Design review of the part shown in the three views and the two pictorial views. Dimensions are in mm from the part's minimum x, y and z. Round coordinates to 2 decimals unless told otherwise and drop trailing zeros. Write each loop counter-clockwise with the first axis right and the second up, starting at its lowest first coordinate (ties: lowest second). Pieces come first, ordered by that corner, then holes. Notation, with made-up numbers: (45, -23.5) -> (90, -23.5) arc R22 cw to (90, -15.5) -> close; hole circle Ø8 at (-21.5, 56.25). An arc over 180 degrees is marked (long way). Answer as a JSON object with one key per item and string values. Group by question number.
1) We need section D-D, the plane x = 56. Write out the cut boundary in (y, z), then the cut area to 3 significant figures.
2) We need section C-C, the plane x = 26.5. Write out the cut boundary in (y, z), then the cut area to 3 significant figures.
3) Insertion check: pin 1 Ø1.6 at (x, z) = (62, 49.5) entering from +Y; pin 2 Ø0.9 at (x, y) = (39, 1) entering from +Z; pin 3 Ø1.5 at (y, z) = (1, 43.5) entering from +X; pin 4 Ø1.5 at (x, y) = (49.5, 1) entering from -Z. Each pin has a flat end and moves straight along its axis. Give the tip position at first contact, or say it passes through.
4) To check wall thickness, follow probe 1 along X at (y, z) = (1.1, 49.5); probe 2 along Z at (x, y) = (28, 1); probe 3 along X at (y, z) = (0.7, 50). State the ranges of each line that lie inside material, in increasing order. Write a range as [from, to].
5) We need section A-A, the plane z = 41. Write out the cut boundary in (x, y), then the cut area to 3 significant figures.
6) We need section B-B, the plane y = 0.65. Write out the cut boundary in (x, z).
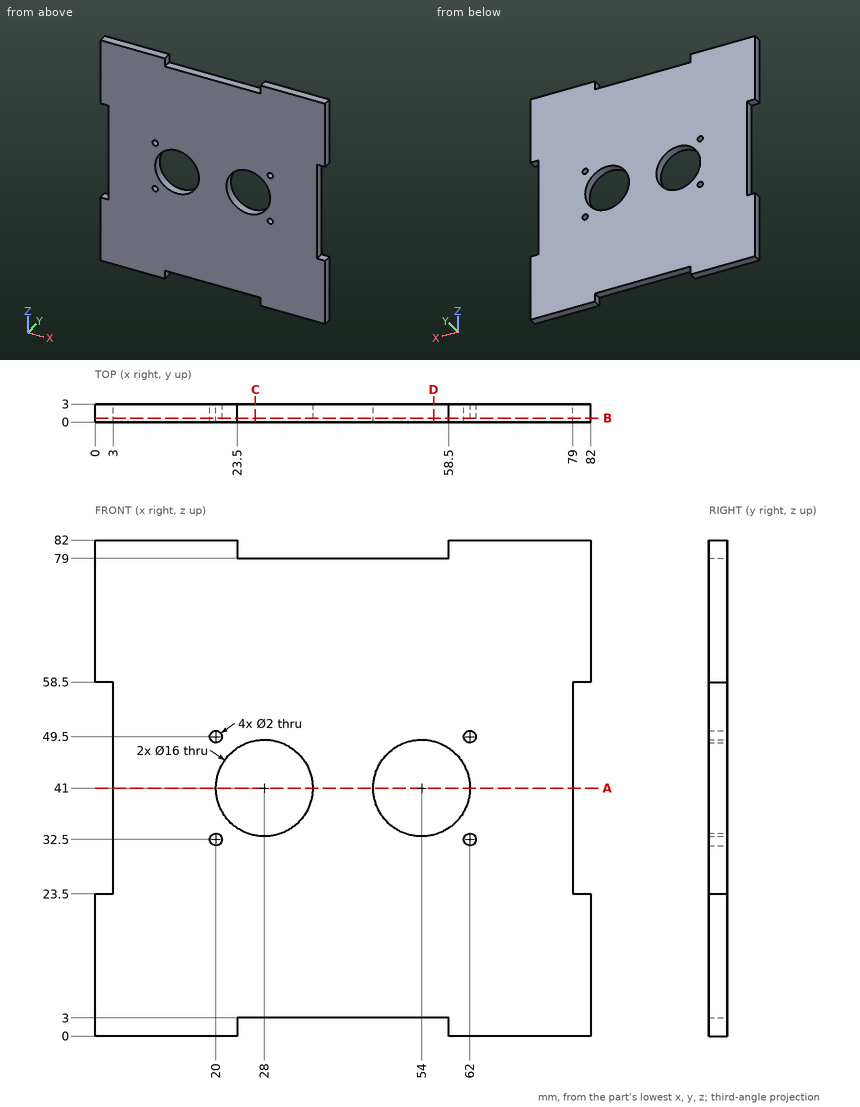
Here are the results:
{
 "1": {"outline": "(0, 3) -> (3, 3) -> (3, 33.25) -> (0, 33.25) -> close; (0, 48.75) -> (3, 48.75) -> (3, 79) -> (0, 79) -> close", "area": "182 mm^2"},
 "2": {"outline": "(0, 3) -> (3, 3) -> (3, 33.14) -> (0, 33.14) -> close; (0, 48.86) -> (3, 48.86) -> (3, 79) -> (0, 79) -> close", "area": "181 mm^2"},
 "3": {"pin 1": "passes through", "pin 2": "stops at z = 79", "pin 3": "stops at x = 79", "pin 4": "stops at z = 3"},
 "4": {"probe 1": "x = [3, 19], [21, 61], [63, 79]", "probe 2": "z = [3, 33], [49, 79]", "probe 3": "x = [3, 19.13], [20.87, 61.13], [62.87, 79]"},
 "5": {"outline": "(3, 0) -> (20, 0) -> (20, 3) -> (3, 3) -> close; (36, 0) -> (46, 0) -> (46, 3) -> (36, 3) -> close; (62, 0) -> (79, 0) -> (79, 3) -> (62, 3) -> close", "area": "132 mm^2"},
 "6": {"outline": "(0, 0) -> (23.5, 0) -> (23.5, 3) -> (58.5, 3) -> (58.5, 0) -> (82, 0) -> (82, 23.5) -> (79, 23.5) -> (79, 58.5) -> (82, 58.5) -> (82, 82) -> (58.5, 82) -> (58.5, 79) -> (23.5, 79) -> (23.5, 82) -> (0, 82) -> (0, 58.5) -> (3, 58.5) -> (3, 23.5) -> (0, 23.5) -> close; hole circle Ø2 at (20, 32.5); hole circle Ø2 at (20, 49.5); hole circle Ø16 at (28, 41); hole circle Ø16 at (54, 41); hole circle Ø2 at (62, 32.5); hole circle Ø2 at (62, 49.5)"}
}
